Work out the finished part from the listing and answer in its coordinate system (mm). Face numbers are marked on the shaded views. Coordinates: 2 decimals unless noted, no trailing zeros. Write each loop counter-clockwise with the first axis right and the second up, starting at its lowest first coordinate (ties: lowest second). Pieces come first, ordered by that corner, then holes. Notation, with made-up numbers: M -13,-34.5 L 20,-34.5 A19 cw 20,-27.5 Z; hole C -5.5,71 d4. An arc over 180 degrees is marked long. Answer as CSV lines item,"result". Start each with the question number.
(1) A cutting plane is placed at B-B on x = -2.75. Give the vertices of the cut face in (y, z), then the cut area to 3 significant figures.
(2) A cutting plane is placed at A-A on y = 176. Give the vertices of the cut face in (x, z).
(3) Flat-ended cylindrical pins translate along their axes: P1, Ø4, axis at x = 6.5, z = -4, coming from the +Y side; P2, Ø7, axis at y = 220, z = 0, coming from the +X side. Find the tip coordinate at first contact, or state that the pin passes through.
(4) A cutting plane is placed at C-C on z = 0. Give the vertices of the cut face in (x, y).
(5) The mould has two halves that part along X. Classify the marked faces 1, 2 and 3: released by +X, released by -X, zero draft, split by the parting line, or undercut.
(6) Find the intervals of material crossed by L1, parallel to Z at x = -3.5, y = 123.5; L2, parallel to Y at x = 8.15, z = 0, in increasing order. Write a range as [from, to].
(7) A cutting plane is placed at D-D on y = 220. Give the vertices of the cut face in (x, z).
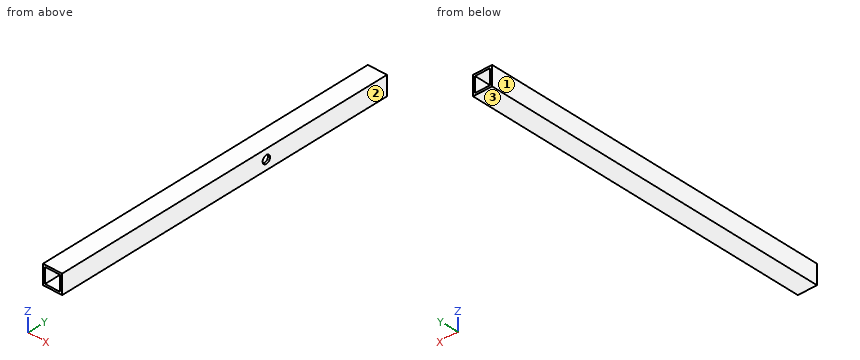
from build123d import *

# Parameters (mm, degrees)
SKETCH1_W           = 19
SKETCH1_H           = 19
SKETCH1_W_2         = 15
SKETCH1_H_2         = 15
EXTRUDE_THIN1_DEPTH = 350
SKETCH2_R           = 4
CUT_EXTRUDE1_DEPTH  = 4


with BuildPart() as part:
    # Sketch1 → Extrude-Thin1 (new body)
    with BuildSketch(Plane(origin=(0, 0, 0), x_dir=(1, 0, 0), z_dir=(0, 1, 0))):
        Rectangle(SKETCH1_W, SKETCH1_H)
        Rectangle(SKETCH1_W_2, SKETCH1_H_2, mode=Mode.SUBTRACT)
    extrude(amount=EXTRUDE_THIN1_DEPTH)

    # Sketch2 → Cut-Extrude1 (cut)
    with BuildSketch(Plane(origin=(9.5, 0, 0), x_dir=(0, 0, -1), z_dir=(1, 0, 0))):
        with Locations((0, 220)):
            Circle(SKETCH2_R)
    extrude(amount=-CUT_EXTRUDE1_DEPTH, mode=Mode.SUBTRACT)


solid = part.part
Here are the results:
1,outline,"M 0,-9.5 L 350,-9.5 L 350,-7.5 L 0,-7.5 Z; M 0,7.5 L 350,7.5 L 350,9.5 L 0,9.5 Z"
1,area,"1,400 mm^2"
2,outline,"M -9.5,-9.5 L 9.5,-9.5 L 9.5,9.5 L -9.5,9.5 Z; hole M -7.5,-7.5 L 7.5,-7.5 L 7.5,7.5 L -7.5,7.5 Z"
3,P1,"stops at y = 350"
3,P2,"stops at x = -7.5"
4,outline,"M -9.5,0 L -7.5,0 L -7.5,350 L -9.5,350 Z; M 7.5,0 L 9.5,0 L 9.5,216 L 7.5,216 Z; M 7.5,224 L 9.5,224 L 9.5,350 L 7.5,350 Z"
5,face 1,"released by -X"
5,face 2,"released by +X"
5,face 3,"zero draft"
6,L1,"z = [-9.5, -7.5], [7.5, 9.5]"
6,L2,"y = [0, 216], [224, 350]"
7,outline,"M -9.5,-9.5 L 9.5,-9.5 L 9.5,-4 L 7.5,-4 L 7.5,-7.5 L -7.5,-7.5 L -7.5,7.5 L 7.5,7.5 L 7.5,4 L 9.5,4 L 9.5,9.5 L -9.5,9.5 Z"
